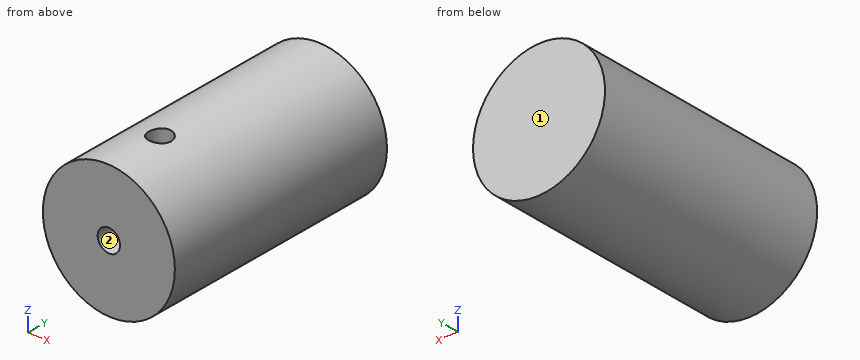
```python
from build123d import *

# Parameters (mm, degrees)
SKETCH1_R           = 37.465
BOSS_EXTRUDE1_DEPTH = 137.16
SKETCH3_R           = 6.35
CUT_EXTRUDE1_DEPTH  = 19.05
SKETCH4_R           = 6.35
CUT_EXTRUDE2_DEPTH  = 19.05


with BuildPart() as part:
    # Sketch1 → Boss-Extrude1 (new body)
    with BuildSketch(Plane(origin=(0, 0, 0), x_dir=(1, 0, 0), z_dir=(0, 1, 0))):
        Circle(SKETCH1_R)
    extrude(amount=BOSS_EXTRUDE1_DEPTH)

    # Sketch3 → Cut-Extrude1 (cut)
    with BuildSketch(Plane.XY.offset(37.465)):
        with Locations((0, 33.02)):
            Circle(SKETCH3_R)
    extrude(amount=-CUT_EXTRUDE1_DEPTH, mode=Mode.SUBTRACT)

    # Sketch4 → Cut-Extrude2 (cut)
    with BuildSketch(Plane.XZ):
        Circle(SKETCH4_R)
    extrude(amount=-CUT_EXTRUDE2_DEPTH, mode=Mode.SUBTRACT)


solid = part.part
```
Check sheet for the modelled part. Datum: model origin and axes. Units: mm. Face numbers are marked on the shaded views. A direction names the side the tool comes from. Give positions to 0.01 mm unless a question says otherwise; leave off trailing zeros. Write each loop counter-clockwise with the first axis right and the second up, starting at its lowest first coordinate (ties: lowest second). Pieces come first, ordered by that corner, then holes. Notation, with made-up numbers: (1.25, -35) - (22.25, -35) arc R16 ccw to (22.25, -26) - close; hole circle Ø3 at (28.5, 4). An arc over 180 degrees is marked (long way). Answer as a JSON object with one key per item and string values. Group by question number.
1) Sectioned sample at B-B (x = 0). Record the cut outline in (y, z) (3 decimals).
2) Thickness scan on probe 1 along X at (y, z) = (8, 0.5); probe 2 along Y at (x, z) = (0, 27.5); probe 3 along Z at (x, y) = (0, 9) (3 decimals). Record the ranges inside material, lowest first. Write a range as from..to.
3) Sectioned sample at A-A (z = -2). Record the cut outline in (x, y).
4) Sectioned sample at C-C (y = 89). Record the cut outline in (x, z) (3 decimals).
5) Depth check by flat-ended pin: P1, Ø1.5, axis at y = 32.5, z = -12, coming from the +X side; P2, Ø5, axis at x = -21, y = 47.5, coming from the +Z side; P3, Ø7.5, axis at x = 0, y = 33.02, coming from the +Z side (3 decimals). Enter the tip coordinate at first touch or a pass-through.
6) Access from +Z, -Z, +X, -X, +Y, -Y to the whole of each face (thin tool, end or side, straight path). Record for the marked faces 1 and 2.
7) Sectioned sample at D-D (z = -24.5). Record the cut outline in (x, y).
Geometry results:
{
 "1": {"outline": "(0, -37.465) - (137.16, -37.465) - (137.16, 37.465) - (39.37, 37.465) - (39.37, 18.415) - (26.67, 18.415) - (26.67, 37.465) - (0, 37.465) - (0, 6.35) - (19.05, 6.35) - (19.05, -6.35) - (0, -6.35) - close"},
 "2": {"probe 1": "x = -37.46..-6.33, 6.33..37.46", "probe 2": "y = 0..26.67, 39.37..137.16", "probe 3": "z = -37.465..-6.35, 6.35..37.465"},
 "3": {"outline": "(-37.41, 0) - (-6.03, 0) - (-6.03, 19.05) - (6.03, 19.05) - (6.03, 0) - (37.41, 0) - (37.41, 137.16) - (-37.41, 137.16) - close"},
 "4": {"outline": "circle Ø74.93 at (0, 0)"},
 "5": {"P1": "stops at x = 35.74", "P2": "stops at z = 32.58", "P3": "stops at z = 18.415"},
 "6": {"face 1": "+Z, -Z, +X, -X, +Y", "face 2": "-Y"},
 "7": {"outline": "(-28.34, 0) - (28.34, 0) - (28.34, 137.16) - (-28.34, 137.16) - close"}
}
